Here's how the part is built. I have some questions about the finished solid (model axes, mm). Coordinates: 2 decimals unless noted, no trailing zeros. Write each loop counter-clockwise with the first axis right and the second up, starting at its lowest first coordinate (ties: lowest second). Pieces come first, ordered by that corner, then holes. Notation, with made-up numbers: (60.5, 27.5) -> (98.5, 27.5) arc R32 cw to (98.5, 57.5) -> close; hole circle Ø4 at (41, 2.25). An arc over 180 degrees is marked (long way). Use a Markdown table: item, result. Add a question column.
```python
from build123d import *

# Parameters (mm, degrees)
SKETCH1_R           = 2.25
BOSS_EXTRUDE1_DEPTH = 5
BOSS_EXTRUDE2_DEPTH = 2


with BuildPart() as part:
    # Sketch1 → Boss-Extrude1 (new body)
    with BuildSketch(Plane.XY):
        with BuildLine():
            Line((-75, 35), (-85, 35))
            ThreePointArc((-85, 35), (-91.25, 28.75), (-85, 22.5))
            Line((-85, 22.5), (-75, 22.5))
            Line((-75, 22.5), (-75, -53.5))
            ThreePointArc((-75, -53.5), (-74.560660172, -54.560660172), (-73.5, -55))
            Line((-73.5, -55), (70, -55))
            ThreePointArc((70, -55), (73.535533906, -53.535533906), (75, -50))
            Line((75, -50), (75, -35))
            Line((75, -35), (85, -35))
            ThreePointArc((85, -35), (91.25, -28.75), (85, -22.5))
            Line((85, -22.5), (75, -22.5))
            Line((75, -22.5), (75, 50))
            ThreePointArc((75, 50), (73.535533906, 53.535533906), (70, 55))
            Line((70, 55), (-70, 55))
            ThreePointArc((-70, 55), (-73.535533906, 53.535533906), (-75, 50))
            Line((-75, 50), (-75, 35))
        make_face()
        with Locations((-85, 28.75)):
            Circle(SKETCH1_R, mode=Mode.SUBTRACT)
        with Locations((85, -28.75)):
            Circle(SKETCH1_R, mode=Mode.SUBTRACT)
    extrude(amount=BOSS_EXTRUDE1_DEPTH)

    # Sketch3 → Boss-Extrude2 (add)
    with BuildSketch(Plane(origin=(0, 0, 0), x_dir=(-1, 0, 0), z_dir=(0, 0, -1))):
        with BuildLine():
            Line((-68.5, -45), (-68.5, 45))
            ThreePointArc((-68.5, 45), (-67.474873734, 47.474873734), (-65, 48.5))
            Line((-65, 48.5), (65, 48.5))
            ThreePointArc((65, 48.5), (67.474873734, 47.474873734), (68.5, 45))
            Line((68.5, 45), (68.5, -45))
            ThreePointArc((68.5, -45), (67.474873734, -47.474873734), (65, -48.5))
            Line((65, -48.5), (-65, -48.5))
            ThreePointArc((-65, -48.5), (-67.474873734, -47.474873734), (-68.5, -45))
        make_face()
    extrude(amount=BOSS_EXTRUDE2_DEPTH)


solid = part.part
```
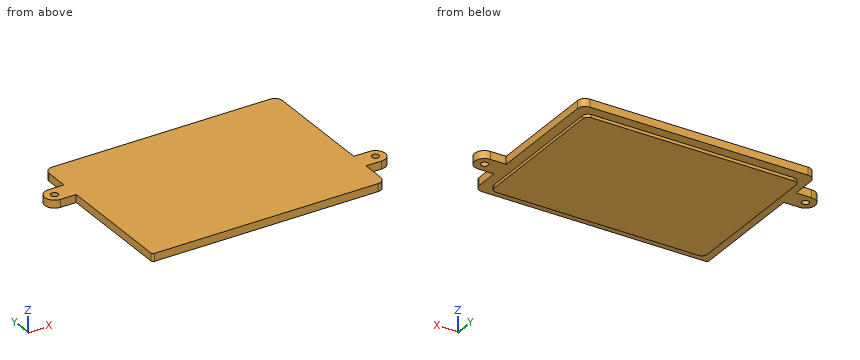
Q1. Please list where these lines run through material, in increasing order: line 1 (Y direction, x = 85, z = 3.9); line 2 (Y direction, x = 15, z = -0.5); line 3 (X direction, y = 38, z = 1.75).
Q2. Suppose I cut it at D-D, the plane x = -80. Write out the boundary of the cut face in (y, z), and give its area (3 significant figures).
Q3. Suppose I cut it at A-A, the plane y = -28.75. Write out the boundary of the cut face in (x, z), and give its area (3 significant figures).
Q4. Suppose I cut it at B-B, the plane x = -48.5. Write out the boundary of the cut face in (y, z).
Q5. Suppose I cut it at C-C, the plane y = -16. Write out the boundary of the cut face in (x, z).
Q6. Will these pins go through, and if not, where does the flat tip stop? pin 1 (2 mm diameter, centred on y = -2.5, z = -1.5, fed in from -X); pin 2 (2.5 mm diameter, centred on y = 2.5, z = 2.5, fed in from -X); pin 3 (1.5 mm diameter, centred on y = -40, z = 1.5, fed in from +X).
Answer key:
| question | item | result |
|---|---|---|
| 1 | line 1 | y = -35 to -31, -26.5 to -22.5 |
| 1 | line 2 | y = -48.5 to 48.5 |
| 1 | line 3 | x = -75 to 75 |
| 2 | outline | (22.5, 0) -> (35, 0) -> (35, 5) -> (22.5, 5) -> close |
| 2 | area | 62.5 mm^2 |
| 3 | outline | (-75, 0) -> (-68.5, 0) -> (-68.5, -2) -> (68.5, -2) -> (68.5, 0) -> (82.75, 0) -> (82.75, 5) -> (-75, 5) -> close; (87.25, 0) -> (91.25, 0) -> (91.25, 5) -> (87.25, 5) -> close |
| 3 | area | 1,080 mm^2 |
| 4 | outline | (-55, 0) -> (-48.5, 0) -> (-48.5, -2) -> (48.5, -2) -> (48.5, 0) -> (55, 0) -> (55, 5) -> (-55, 5) -> close |
| 5 | outline | (-75, 0) -> (-68.5, 0) -> (-68.5, -2) -> (68.5, -2) -> (68.5, 0) -> (75, 0) -> (75, 5) -> (-75, 5) -> close |
| 6 | pin 1 | stops at x = -68.5 |
| 6 | pin 2 | stops at x = -75 |
| 6 | pin 3 | stops at x = 75 |
